Source: CAD feature listing. Evaluate the final solid. Frame: model axes, mm. Face numbers are marked on the shaded views. A direction names the side the tool comes from. Round coordinates to 2 decimals unless told otherwise and drop trailing zeros. Write each loop counter-clockwise with the first axis right and the second up, starting at its lowest first coordinate (ties: lowest second). Pieces come first, ordered by that corner, then holes. Notation, with made-up numbers: M -37,-31.5 L 22,-31.5 A24 cw 22,-6.5 Z; hole C -3.5,-12.5 d6. An arc over 180 degrees is marked long. Answer in a Markdown table with one row per item. Add a question column.
Item 1: Contact query for flat-ended pins moving along their axis: pin 1 (2 mm diameter, centred on x = -2, z = 4, fed in from -Y); pin 2 (4 mm diameter, centred on x = 7, y = 1, fed in from +Z); pin 3 (2 mm diameter, centred on y = 2, z = 4.5, fed in from +X); pin 4 (3 mm diameter, centred on x = 7, z = 0, fed in from +Y). Output: stop coordinate, or through.
Item 2: Mould query, pull axis Z, two halves, no side actions, for the marked faces 1, 2 and 3. Classes: released by +Z, released by -Z, zero draft, split by the parting line, or undercut.
Item 3: Cut plane A-A on y = 5.5. Return loops of the section in (x, z).
Item 4: Material intervals for probe 1 along Z at (x, y) = (-3.5, 6.5); probe 2 along Y at (x, z) = (5, -2.75); probe 3 along Z at (x, y) = (6, 0.5), sorted ascending.
Item 5: Cut plane B-B on y = 3.25. Return loops of the section in (x, z), and give its area (3 significant figures).
Item 6: Set-up query: the marked faces 4 and 5. Return all of +Z, -Z, +X, -X, +Y, -Y with unobstructed straight access to the full face (end or side cutting, diameter ignored); none if empty.
from build123d import *

# Parameters (mm, degrees)
F2_R      = 0.5
F5_DEPTH  = 5
F6_R      = 0.5
F7_R      = 2
F8_DEPTH  = 7
F9_R      = 1.2
F10_DEPTH = 25


with BuildPart() as f1:
    # F0 (on Top) → F1 (revolve)
    with BuildSketch(Plane.XY):
        with BuildLine():
            Line((0, 9), (0, 0))
            Line((0, 0), (11, 0))
            Line((11, 0), (11, 4))
            Line((11, 4), (10.5, 7))
            ThreePointArc((10.5, 7), (10.0017468007, 7.1915925315), (9.5, 7.3738398822))
            Line((9.5, 7.3738398822), (9.5, 6.5449972332))
            Line((9.5, 6.5449972332), (9, 6.5449972332))
            Line((9, 6.5449972332), (9, 7.5449972332))
            ThreePointArc((9, 7.5449972332), (4.5584271698, 8.6339031037), (0, 9))
        make_face()
    revolve(axis=Axis((0, 4.5, 0), (0, -1, 0)))

    # F2
    f2_edges = [f1.edges().sort_by_distance(p)[0] for p in [
        (-10.5, 7, 0),
    ]]
    fillet(f2_edges, radius=F2_R)

    # F4 (on offset) → F5 (cut)
    with BuildSketch(Plane.XZ.offset(-9)):
        with BuildLine():
            ThreePointArc((-4.905379299, -6.3195928613), (5.6568542495, -5.6568542495), (6.3195928613, 4.905379299))
            Line((6.3195928613, 4.905379299), (-4.905379299, -6.3195928613))
        make_face()
        with BuildLine():
            Line((-6.3195928613, -4.905379299), (4.905379299, 6.3195928613))
            ThreePointArc((4.905379299, 6.3195928613), (-5.6568542495, 5.6568542495), (-6.3195928613, -4.905379299))
        make_face()
    extrude(amount=F5_DEPTH, mode=Mode.SUBTRACT)

    # F6
    f6_edges = [f1.edges().sort_by_distance(p)[0] for p in [
        (6.319593, 5.928385, 4.905379),
        (-4.905379, 5.928385, -6.319593),
        (-6.319593, 5.928385, -4.905379),
        (4.905379, 5.928385, 6.319593),
    ]]
    fillet(f6_edges, radius=F6_R)

    # F7 (on offset) → F8 (cut)
    with BuildSketch(Plane.XZ.offset(-9)):
        with Locations((6, 0)):
            Circle(F7_R)
        with Locations((-6, 0)):
            Circle(F7_R)
    extrude(amount=F8_DEPTH, mode=Mode.SUBTRACT)

    # F9 (on face) → F10 (cut)
    with BuildSketch(Plane(origin=(0, 2, 0), x_dir=(-1, 0, 0), z_dir=(0, 1, 0))):
        with Locations((-6, 0)):
            Circle(F9_R)
        with Locations((6, 0)):
            Circle(F9_R)
    extrude(amount=-F10_DEPTH, mode=Mode.SUBTRACT)


solid = f1.part
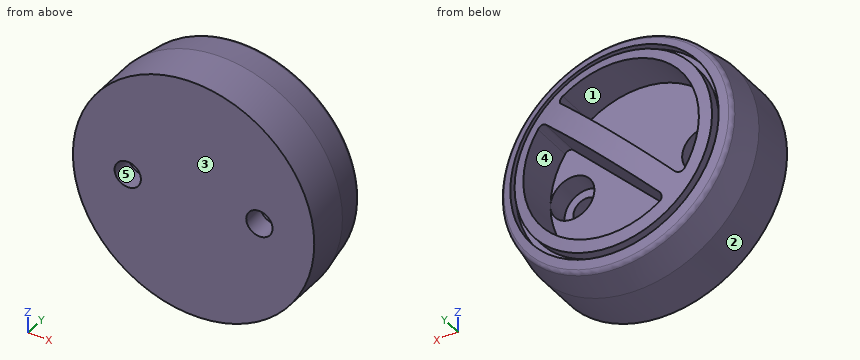
Results below:
| question | item | result |
|---|---|---|
| 1 | pin 1 | y = 0 |
| 1 | pin 2 | z = 9.8 |
| 1 | pin 3 | x = 10.43 |
| 1 | pin 4 | y = 7.86 |
| 2 | face 1 | undercut |
| 2 | face 2 | split by the parting line |
| 2 | face 3 | zero draft |
| 3 | outline | C 0,0 d21.5; hole M -6.67,-4.41 A0.5 ccw -5.9,-4.49 L 4.49,5.9 A0.5 ccw 4.41,6.67 A8 ccw Z; hole M -4.49,-5.9 A0.5 ccw -4.41,-6.67 A8 ccw 6.67,4.41 A0.5 ccw 5.9,4.49 Z |
| 4 | probe 1 | -9.99 to -7.19, -4.91 to -2.09, 7.19 to 9.99 |
| 4 | probe 2 | 0 to 4 |
| 4 | probe 3 | -9.22 to -1.2, 1.2 to 9.22 |
| 5 | outline | C 0,0 d22; hole C -6,0 d4; hole C 6,0 d4 |
| 5 | area | 355 mm2 |
| 6 | face 4 | +Y |
| 6 | face 5 | +Y, -Y |
